from build123d import *

# Parameters (mm, degrees)
BOSS_EXTRUDE1_DEPTH        = 1.6002
SKETCH2_R                  = 38.1
CUT_EXTRUDE1_DEPTH         = 2.6002
CIRPATTERN1_COUNT          = 8
F_10_CLEARANCE_HOLE1_D     = 5.6134
F_10_CLEARANCE_HOLE1_DEPTH = 9.53
F_10_CLEARANCE_HOLE1_TIP   = 1.686435499


with BuildPart() as part:
    # Sketch1 → Boss-Extrude1 (new body)
    with BuildSketch(Plane.XY):
        Polygon((161.3627, -107.93570835), (59.7625, -107.93570835), (59.7625, -153.41070835), (-161.3627, -153.41070835), (-161.3627, 145.48590835), (161.3627, 145.48590835), align=None)
    extrude(amount=BOSS_EXTRUDE1_DEPTH)

    # Sketch2 → Cut-Extrude1 (cut, through all)
    with BuildSketch(Plane.XY.offset(1.6002)):
        with Locations((-93.3627, 0)):
            Circle(SKETCH2_R)
    extrude(amount=-CUT_EXTRUDE1_DEPTH, mode=Mode.SUBTRACT)

    # Sketch11 → #4 Clearance Hole1 (revolve, cut)
    with BuildSketch(Plane(origin=(-93.3627, 50.8, 1.6002), x_dir=(0, -1, 0), z_dir=(1, 0, 0))):
        Polygon((0, 0), (0, 173.855187864), (1.4732, 172.97), (1.4732, 0), align=None)
    f_4_clearance_hole1 = revolve(axis=Axis((-93.3627, 50.8, 7.9502), (0, 0, -1)), mode=Mode.SUBTRACT)

    # CirPattern1: #4 Clearance Hole1 ×8 about axis
    cirpattern1_axis = Axis((-93.3627, 0, 0), (0, 0, 1))
    for i in range(1, CIRPATTERN1_COUNT):
        add(f_4_clearance_hole1.rotate(cirpattern1_axis, i * 360 / CIRPATTERN1_COUNT), mode=Mode.SUBTRACT)

    # #10 Clearance Hole1
    with Locations(Plane.XY.offset(1.6002)):
        with Locations((-155, 105.78570835), (-155, 0), (-155, -105.78570835), (155, 105.78570835), (155, 25.27849165)):
            Hole(F_10_CLEARANCE_HOLE1_D / 2, depth=F_10_CLEARANCE_HOLE1_DEPTH)
            with Locations((0, 0, -(F_10_CLEARANCE_HOLE1_DEPTH + F_10_CLEARANCE_HOLE1_TIP / 2))):  # 118° drill point
                Cone(0, F_10_CLEARANCE_HOLE1_D / 2, F_10_CLEARANCE_HOLE1_TIP, mode=Mode.SUBTRACT)


solid = part.part
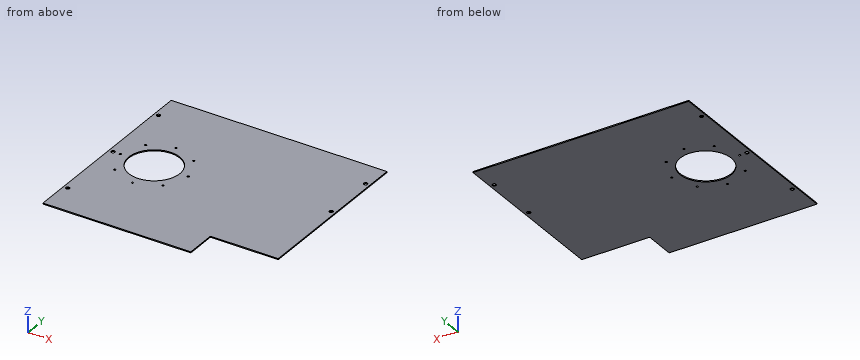
Check sheet for the modelled part. Datum: model origin and axes. Units: mm. Round coordinates to 2 decimals unless told otherwise and drop trailing zeros. Loops run counter-clockwise (first coordinate to the right, second up) from the corner with the lowest first, then second, coordinate; pieces in that order, holes last.
1. Gauge pin test, flat end, axial feed: pin 1 Ø2.5 at (x, y) = (-57.44, 35.92) entering from +Z. Record the tip position at first contact, or that the pin passes through.
2. Sectioned sample at A-A on x = -64. Record the boundary of the cut face in (y, z).
3. Scan lines: probe 1 along Y at (x, z) = (-94, 0.25); probe 2 along Y at (x, z) = (-128, 0.55); probe 3 along Y at (x, z) = (-87.5, 1.25). Record each from-to range of solid material in increasing order.
4. Sectioned sample at B-B on z = 0.35. Give the number of separate pieces and of enclosed holes in the cut face, and give its area (3 significant figures).
5. Sectioned sample at C-C on x = 116. Record the boundary of the cut face in (y, z), and give its area (3 significant figures).
Recorded:
1. pin 1: passes through
2. outline: (-153.41, 0) - (-24.28, 0) - (-24.28, 1.6) - (-153.41, 1.6) - close; (24.28, 0) - (145.49, 0) - (145.49, 1.6) - (24.28, 1.6) - close
3. probe 1: y = -153.41 to -52.13, -49.47 to -38.09, 38.09 to 49.47, 52.13 to 145.49
3. probe 2: y = -153.41 to -36.64, -35.2 to -15.87, 15.87 to 35.2, 36.64 to 145.49
3. probe 3: y = -153.41 to -37.65, 37.65 to 145.49
4. separate pieces: 1
4. enclosed holes: 14
4. area: 87,100 mm2
5. outline: (-107.94, 0) - (145.49, 0) - (145.49, 1.6) - (-107.94, 1.6) - close
5. area: 406 mm2
